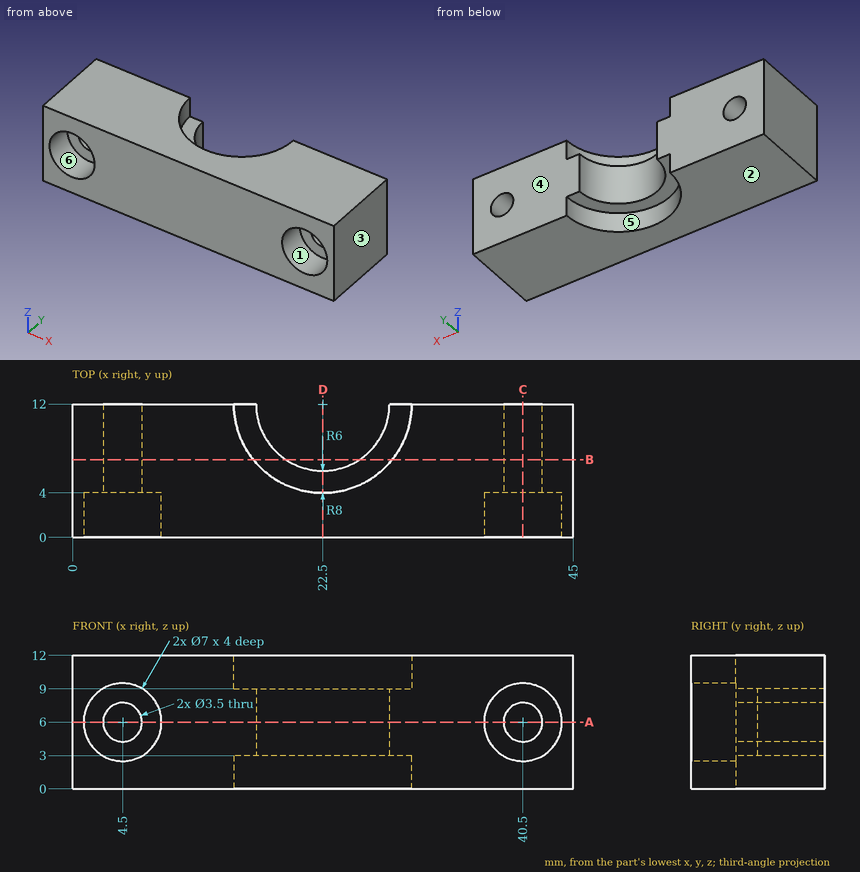
Drawing for the job (mm, zero at the part's lowest x, y, z). A direction names the side the tool comes from. Round coordinates to 2 decimals unless told otherwise and drop trailing zeros. Loops run counter-clockwise (first coordinate to the right, second up) from the corner with the lowest first, then second, coordinate; pieces in that order, holes last. Notation, with made-up numbers: (19, 84) - (24, 84) arc R4 ccw to (24, 90) - close; hole circle Ø11 at (28.25, 82). An arc over 180 degrees is marked (long way). Return JSON: item names as keys, results as strings. Group by question number.
Q1. Flat gauge pins, fed straight in: pin 1 Ø1 at (x, y) = (29, 8.5) entering from +Z; pin 2 Ø3 at (x, z) = (4.5, 6) entering from +Y. Where does each tip first touch, or does it go through?
Q2. Band-saw the part on D-D on x = 22.5. Give the cut face in (y, z).
Q3. Drill centre lines: line 1 along Z through (x, y) = (40.5, 9.25); line 2 along Z through (x, y) = (40.5, 3.1); line 3 along X through (y, z) = (7, 6.25). Where is each one in solid material? Low to high. Write a range as [from, to].
Q4. Band-saw the part on B-B on y = 7. Give the cut face in (x, z) (3 decimals).
Q5. Band-saw the part on A-A on z = 6. Give the cut face in (x, y), plus the area to 3 significant figures.
Q6. Tool access for the marked faces 4, 5 and 6: list every direction of +Z, -Z, +X, -X, +Y, -Y with a clear straight run to the whole face (end or side of a thin tool).
Q7. Band-saw the part on C-C on x = 40.5. Give the cut face in (y, z).
Q8. Two-plate mould, pull along Z, no slides. Class the marked faces 1, 2 and 3: +Z half, -Z half, draft (parallel to the pull), parting line (faces both ways), or undercut.
Solutions:
{
 "1": {"pin 1": "stops at z = 9", "pin 2": "passes through"},
 "2": {"outline": "(0, 0) - (4, 0) - (4, 3) - (6, 3) - (6, 9) - (4, 9) - (4, 12) - (0, 12) - close"},
 "3": {"line 1": "z = [0, 4.25], [7.75, 12]", "line 2": "z = [0, 2.5], [9.5, 12]", "line 3": "x = [0, 2.77], [6.23, 19.18], [25.82, 38.77], [42.23, 45]"},
 "4": {"outline": "(0, 0) - (16.255, 0) - (16.255, 3) - (19.183, 3) - (19.183, 9) - (16.255, 9) - (16.255, 12) - (0, 12) - close; (25.817, 3) - (28.745, 3) - (28.745, 0) - (45, 0) - (45, 12) - (28.745, 12) - (28.745, 9) - (25.817, 9) - close; hole circle Ø3.5 at (4.5, 6); hole circle Ø3.5 at (40.5, 6)"},
 "5": {"outline": "(0, 0) - (1, 0) - (1, 4) - (2.75, 4) - (2.75, 12) - (0, 12) - close; (6.25, 4) - (8, 4) - (8, 0) - (37, 0) - (37, 4) - (38.75, 4) - (38.75, 12) - (28.5, 12) arc R6 cw to (16.5, 12) - (6.25, 12) - close; (42.25, 4) - (44, 4) - (44, 0) - (45, 0) - (45, 12) - (42.25, 12) - close", "area": "371 mm^2"},
 "6": {"face 4": "+Z, -Z, +X, -X, +Y", "face 5": "-Z, +Y", "face 6": "-Y"},
 "7": {"outline": "(0, 0) - (12, 0) - (12, 4.25) - (4, 4.25) - (4, 2.5) - (0, 2.5) - close; (0, 9.5) - (4, 9.5) - (4, 7.75) - (12, 7.75) - (12, 12) - (0, 12) - close"},
 "8": {"face 1": "undercut", "face 2": "-Z half", "face 3": "draft"}
}
